Verification items for the finished model (mm, model axes). Give positions to 0.01 mm unless a question says otherwise; leave off trailing zeros. Answer as a JSON object with one key per item and string values. Group by question number.
(1) Section check A-A (y = 0.8). Count the separate pieces of the cut face and the enclosed holes in it, then the cut area to 3 significant figures.
(2) Mould release check, pull along X, two halves, no side actions. Record for faces 1 (the face through (28, 1.588, 130)), 2 (the face through (171, 0, 67)), 3 (the face through (182, 0, 56)), 4 (the face through (-121.246, -0.022, 254.366)): +X half, -X half, draft (parallel to the pull), parting line (faces both ways), or undercut.
(3) Thickness scan on line 1 (X direction, y = 1.25, z = 83); line 2 (X direction, y = 0.6, z = 127); line 3 (X direction, y = -0.4, z = 135.5). Record the ranges inside material, lowest first.
(4) Depth check by flat-ended pin: pin 1 Ø4 at (x, z) = (172.54, 242.09) entering from +Y; pin 2 Ø16 at (x, z) = (172.49, 137.77) entering from +Y; pin 3 Ø1 at (y, z) = (0.5, -2) entering from -X (3 decimals); pin 4 Ø1.6 at (x, y) = (204.5, -0.5) entering from -Z. Enter the tip coordinate at first touch or a pass-through.
```python
from build123d import *

# Parameters (mm, degrees)
SKETCH1_W            = 308.08168
SKETCH1_H            = 3.175
BOSS_EXTRUDE1_DEPTH  = 267.83
SKETCH3_W            = 267.83
SKETCH3_H            = 3.175
BOSS_EXTRUDE3_DEPTH  = 3.175
SKETCH4_W            = 50.8889
SKETCH4_H            = 3.175
BOSS_EXTRUDE4_DEPTH  = 267.83
CUT_EXTRUDE1_DEPTH   = 340.191055801
SKETCH17_W           = 267.83
SKETCH17_H           = 3.175
BOSS_EXTRUDE5_DEPTH  = 3.175
CUT_EXTRUDE3_DEPTH   = 340.191055801
SKETCH25_R           = 3.175
CUT_EXTRUDE8_DEPTH   = 3.175
SKETCH27_R           = 5
CUT_EXTRUDE9_DEPTH   = 340.191055801
SKETCH31_R           = 1.5875
CUT_EXTRUDE10_DEPTH  = 340.191055801
LPATTERN1_COUNT      = 3
LPATTERN1_PITCH      = 58
M4_CLEARANCE_HOLE1_D = 4.8
SKETCH36_W           = 57.15
SKETCH36_H           = 3.175
SKETCH36_W_2         = 26.9875
BOSS_EXTRUDE6_DEPTH  = 3.175
SKETCH37_W           = 3.175
SKETCH37_H           = 124.4419914
CUT_EXTRUDE11_DEPTH  = 340.191055801
SKETCH38_W           = 3.175
SKETCH38_H           = 146.0243
CUT_EXTRUDE12_DEPTH  = 340.191055801
SKETCH39_W           = 6.35
SKETCH39_H           = 9.525
CUT_EXTRUDE13_DEPTH  = 340.191055801
SKETCH40_R           = 6.25
CUT_EXTRUDE14_DEPTH  = 340.191055801


with BuildPart() as part:
    # Sketch1 → Boss-Extrude1 (new body)
    with BuildSketch(Plane.XY):
        Rectangle(SKETCH1_W, SKETCH1_H)
    extrude(amount=BOSS_EXTRUDE1_DEPTH)

    # Sketch3 → Boss-Extrude3 (add)
    with BuildSketch(Plane(origin=(154.04084, 0, 0), x_dir=(0, 0, -1), z_dir=(1, 0, 0))):
        with Locations((-133.915, 0)):
            Rectangle(SKETCH3_W, SKETCH3_H)
    extrude(amount=BOSS_EXTRUDE3_DEPTH)

    # Sketch4 → Boss-Extrude4 (add)
    with BuildSketch(Plane.XY.offset(267.83)):
        with Locations((182.66029, 0)):
            Rectangle(SKETCH4_W, SKETCH4_H)
    extrude(amount=-BOSS_EXTRUDE4_DEPTH)

    # Sketch6 → Cut-Extrude1 (cut, through all)
    with BuildSketch(Plane(origin=(0, 1.5875, 0), x_dir=(1, 0, 0), z_dir=(0, 1, 0))):
        Polygon((208.10474, -240.606362049), (106.50474, -267.83), (208.10474, -267.83), align=None)
    extrude(amount=-CUT_EXTRUDE1_DEPTH, mode=Mode.SUBTRACT)

    # Sketch17 → Boss-Extrude5 (add)
    with BuildSketch(Plane.ZY.offset(154.04084)):
        with Locations((133.915, 0)):
            Rectangle(SKETCH17_W, SKETCH17_H)
    extrude(amount=BOSS_EXTRUDE5_DEPTH)

    # Sketch11 → Cut-Extrude3 (cut, through all)
    with BuildSketch(Plane.XZ.offset(1.5875)):
        Polygon((-157.21584, 241.2743), (-84.254653892, 267.83), (-157.21584, 267.83), align=None)
    extrude(amount=-CUT_EXTRUDE3_DEPTH, mode=Mode.SUBTRACT)

    # Sketch25 → Cut-Extrude8 (cut)
    with BuildSketch(Plane.XZ.offset(1.5875)):
        with Locations(Location((-115.322188641, 247.921359373, 0), (0, 0, 270))):
            Circle(SKETCH25_R)
        with Locations(Location((-50.97526, 258.94, 0), (0, 0, 270))):
            Circle(SKETCH25_R)
        with Locations(Location((11.25474, 258.94, 0), (0, 0, 270))):
            Circle(SKETCH25_R)
        with Locations(Location((73.48474, 258.94, 0), (0, 0, 270))):
            Circle(SKETCH25_R)
        with Locations(Location((172.54474, 242.09298883, 0), (0, 0, 270))):
            Circle(SKETCH25_R)
        with Locations(Location((131.90474, 252.982444011, 0), (0, 0, 270))):
            Circle(SKETCH25_R)
    extrude(amount=-CUT_EXTRUDE8_DEPTH, mode=Mode.SUBTRACT)

    # Sketch27 → Cut-Extrude9 (cut, through all)
    with BuildSketch(Plane.XZ.offset(1.5875)):
        with Locations(Location((172.48674, 137.774823778, 0), (0, 0, 270))):
            Circle(SKETCH27_R)
        with Locations(Location((183.48674, 137.774823778, 0), (0, 0, 270))):
            Circle(SKETCH27_R)
        with Locations(Location((194.48674, 137.774823778, 0), (0, 0, 270))):
            Circle(SKETCH27_R)
        with Locations(Location((194.48674, 126.774823778, 0), (0, 0, 270))):
            Circle(SKETCH27_R)
        with Locations(Location((194.48674, 115.774823778, 0), (0, 0, 270))):
            Circle(SKETCH27_R)
        with Locations(Location((183.48674, 126.774823778, 0), (0, 0, 270))):
            Circle(SKETCH27_R)
        with Locations(Location((183.48674, 115.774823778, 0), (0, 0, 270))):
            Circle(SKETCH27_R)
        with Locations(Location((172.48674, 115.774823778, 0), (0, 0, 270))):
            Circle(SKETCH27_R)
        with Locations(Location((172.48674, 126.774823778, 0), (0, 0, 270))):
            Circle(SKETCH27_R)
        with Locations(Location((194.48674, 71.774823778, 0), (0, 0, 270))):
            Circle(SKETCH27_R)
        with Locations(Location((194.48674, 60.774823778, 0), (0, 0, 270))):
            Circle(SKETCH27_R)
        with Locations(Location((194.48674, 49.774823778, 0), (0, 0, 270))):
            Circle(SKETCH27_R)
        with Locations(Location((183.48674, 71.774823778, 0), (0, 0, 270))):
            Circle(SKETCH27_R)
        with Locations(Location((183.48674, 60.774823778, 0), (0, 0, 270))):
            Circle(SKETCH27_R)
        with Locations(Location((183.48674, 49.774823778, 0), (0, 0, 270))):
            Circle(SKETCH27_R)
        with Locations(Location((172.48674, 49.774823778, 0), (0, 0, 270))):
            Circle(SKETCH27_R)
        with Locations(Location((172.48674, 60.774823778, 0), (0, 0, 270))):
            Circle(SKETCH27_R)
        with Locations(Location((172.48674, 71.774823778, 0), (0, 0, 270))):
            Circle(SKETCH27_R)
    extrude(amount=-CUT_EXTRUDE9_DEPTH, mode=Mode.SUBTRACT)

    # Sketch31 → Cut-Extrude10 (cut, symmetric)
    with BuildSketch(Plane.XZ.offset(1.5875)):
        with Locations(Location((183.48674, 151.774823778, 0), (0, 0, 270))):
            Circle(SKETCH31_R)
    cut_extrude10 = extrude(amount=CUT_EXTRUDE10_DEPTH, both=True, mode=Mode.SUBTRACT)

    # LPattern1: Cut-Extrude10 ×3
    with Locations(*[(0, 0, -i * LPATTERN1_PITCH) for i in range(1, LPATTERN1_COUNT)]):
        add(cut_extrude10, mode=Mode.SUBTRACT)

    # M4 Clearance Hole1 (through all)
    with Locations(Plane.XZ.offset(1.5875)):
        with Locations((180.96500002, 176.776), (-97.77095, 213.2849914), (3.82905, 213.2849914), (105.42905, 213.2849914)):
            Hole(M4_CLEARANCE_HOLE1_D / 2)

    # Sketch36 → Boss-Extrude6 (add)
    with BuildSketch(Plane(origin=(0, 0, 0), x_dir=(-1, 0, 0), z_dir=(0, 0, -1))):
        Rectangle(SKETCH36_W, SKETCH36_H)
        with Locations((-182.66100002, 0)):
            Rectangle(SKETCH36_W_2, SKETCH36_H)
    extrude(amount=BOSS_EXTRUDE6_DEPTH)

    # Sketch37 → Cut-Extrude11 (cut, through all)
    with BuildSketch(Plane.XZ.offset(1.5875)):
        with Locations((155.62850002, 62.2209957)):
            Rectangle(SKETCH37_W, SKETCH37_H)
    extrude(amount=-CUT_EXTRUDE11_DEPTH, mode=Mode.SUBTRACT)

    # Sketch38 → Cut-Extrude12 (cut, through all)
    with BuildSketch(Plane.XZ.offset(1.5875)):
        with Locations((-155.62834, 73.01215)):
            Rectangle(SKETCH38_W, SKETCH38_H)
    extrude(amount=-CUT_EXTRUDE12_DEPTH, mode=Mode.SUBTRACT)

    # Sketch39 → Cut-Extrude13 (cut, through all)
    with BuildSketch(Plane.XZ.offset(1.5875)):
        with Locations((204.92974, 93.774823778)):
            Rectangle(SKETCH39_W, SKETCH39_H)
        with Locations((204.92974, 201.724823778)):
            Rectangle(SKETCH39_W, SKETCH39_H)
    extrude(amount=-CUT_EXTRUDE13_DEPTH, mode=Mode.SUBTRACT)

    # Sketch40 → Cut-Extrude14 (cut, through all)
    with BuildSketch(Plane.XZ.offset(1.5875)):
        with Locations(Location((182.66100002, 196.101, 0), (0, 0, 270))):
            Circle(SKETCH40_R)
    extrude(amount=-CUT_EXTRUDE14_DEPTH, mode=Mode.SUBTRACT)


solid = part.part
```
Solutions:
{
 "1": {"separate pieces": "1", "enclosed holes": "32", "area": "93,000 mm2"},
 "2": {"face 1": "draft", "face 2": "undercut", "face 3": "undercut", "face 4": "-X half"},
 "3": {"line 1": "x = -154.04 to 154.04, 157.22 to 208.1", "line 2": "x = -154.04 to 167.49, 177.48 to 178.49, 188.48 to 189.49, 199.48 to 208.1", "line 3": "x = -154.04 to 168.03, 176.94 to 179.03, 187.94 to 190.03, 198.94 to 208.1"},
 "4": {"pin 1": "passes through", "pin 2": "stops at y = 1.59", "pin 3": "stops at x = -28.575", "pin 4": "stops at z = 0"}
}
